Design review of the part built by this model. Coordinates are the model's own, in mm. Face numbers are marked on the shaded views. A direction names the side the tool comes from. Give positions to 0.01 mm unless a question says otherwise; leave off trailing zeros. Order: outer loops, then holes, each group sorted by start corner. A loop starts at its lowest first (then second) coordinate and runs counter-clockwise, first axis right, second up. Notation, with made-up numbers: M 78,-18.5 L 88,-18.5 A10 cw 88,-4.5 Z; hole C 23.5,-16.75 d2. An arc over 180 degrees is marked long. Answer as a JSON object with one key per item and string values.
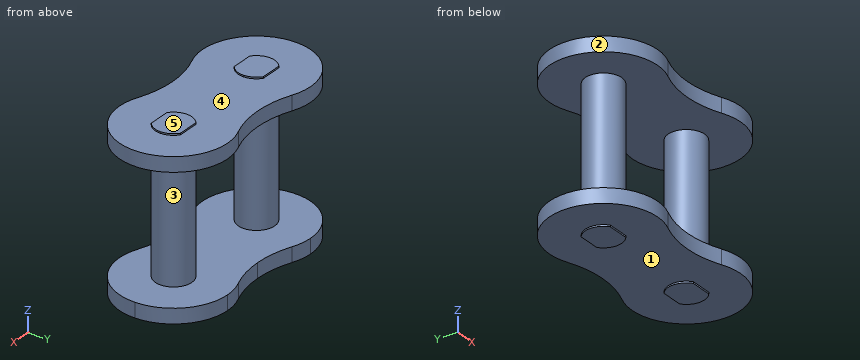
from build123d import *

# Parameters (mm, degrees)
SKETCH1_R           = 2.9718
BOSS_EXTRUDE1_DEPTH = 2.3876
SKETCH2_R           = 2.9718
BOSS_EXTRUDE2_DEPTH = 25.4
BOSS_EXTRUDE3_START = -2.3876
BOSS_EXTRUDE3_DEPTH = 2.3876
BOSS_EXTRUDE4_DEPTH = 0.254


with BuildPart() as part:
    # Sketch1 → Boss-Extrude1 (new body)
    # profile 1 of 12: a face of its own
    with BuildSketch(Plane.XY):
        with BuildLine():
            Line((-5.1181, 4.4069), (-9.525, 8.8138))
            ThreePointArc((-9.525, 8.8138), (-18.169445304, -1.71948708), (-6.152104764, -8.142889424))
            ThreePointArc((-6.152104764, -8.142889424), (-2.196593131, -4.89668492), (-0.7112, 0))
            Line((-0.7112, 0), (-5.1181, 4.4069))
        make_face()
        with Locations((-9.525, 0)):
            Circle(SKETCH1_R, mode=Mode.SUBTRACT)
    # profile 2 of 12: a face of its own
    with BuildSketch(Plane.XY):
        with BuildLine():
            ThreePointArc((-6.152104764, 8.142889424), (-7.80551292, 8.644445304), (-9.525, 8.8138))
            Line((-9.525, 8.8138), (-5.1181, 4.4069))
            Line((-5.1181, 4.4069), (-3.292702252, 6.232297748))
            ThreePointArc((-3.292702252, 6.232297748), (-4.62831508, 7.328406869), (-6.152104764, 8.142889424))
        make_face()
    # profile 3 of 12: a face of its own
    with BuildSketch(Plane.XY):
        with BuildLine():
            Line((-3.292702252, 6.232297748), (-5.1181, 4.4069))
            Line((-5.1181, 4.4069), (-0.7112, 0))
            ThreePointArc((-0.7112, 0), (-1.382110576, 3.372895236), (-3.292702252, 6.232297748))
        make_face()
    # profile 4 of 12: a face of its own
    with BuildSketch(Plane.XY):
        with BuildLine():
            ThreePointArc((-3.292702252, 6.232297748), (-1.382110576, 3.372895236), (-0.7112, 0))
            Line((-0.7112, 0), (0.7112, 0))
            ThreePointArc((0.7112, 0), (1.382110576, 3.372895236), (3.292702252, 6.232297748))
            Line((3.292702252, 6.232297748), (0, 6.232297748))
            Line((0, 6.232297748), (-3.292702252, 6.232297748))
        make_face()
    # profile 5 of 12: a face of its own
    with BuildSketch(Plane.XY):
        with BuildLine():
            ThreePointArc((-0.7112, 0), (-2.196593131, -4.89668492), (-6.152104764, -8.142889424))
            ThreePointArc((-6.152104764, -8.142889424), (0, -6.944339829), (6.152104764, -8.142889424))
            ThreePointArc((6.152104764, -8.142889424), (2.196593131, -4.89668492), (0.7112, 0))
            Line((0.7112, 0), (-0.7112, 0))
        make_face()
    # profile 6 of 12: a face of its own
    with BuildSketch(Plane.XY):
        with BuildLine():
            ThreePointArc((18.3388, 0), (15.757297748, 6.232297748), (9.525, 8.8138))
            Line((9.525, 8.8138), (5.1181, 4.4069))
            Line((5.1181, 4.4069), (0.7112, 0))
            ThreePointArc((0.7112, 0), (2.196593131, -4.89668492), (6.152104764, -8.142889424))
            ThreePointArc((6.152104764, -8.142889424), (14.42168492, -7.328406869), (18.3388, 0))
        make_face()
        with Locations((9.525, 0)):
            Circle(SKETCH1_R, mode=Mode.SUBTRACT)
    # profile 7 of 12: a face of its own
    with BuildSketch(Plane.XY):
        with BuildLine():
            Line((5.1181, 4.4069), (9.525, 8.8138))
            ThreePointArc((9.525, 8.8138), (7.80551292, 8.644445304), (6.152104764, 8.142889424))
            ThreePointArc((6.152104764, 8.142889424), (4.62831508, 7.328406869), (3.292702252, 6.232297748))
            Line((3.292702252, 6.232297748), (5.1181, 4.4069))
        make_face()
    # profile 8 of 12: a face of its own
    with BuildSketch(Plane.XY):
        with BuildLine():
            Line((0.7112, 0), (5.1181, 4.4069))
            Line((5.1181, 4.4069), (3.292702252, 6.232297748))
            ThreePointArc((3.292702252, 6.232297748), (1.382110576, 3.372895236), (0.7112, 0))
        make_face()
    # profile 9 of 12: a face of its own
    with BuildSketch(Plane.XY):
        with BuildLine():
            Line((5.1181, 4.4069), (9.525, 8.8138))
            ThreePointArc((9.525, 8.8138), (7.80551292, 8.644445304), (6.152104764, 8.142889424))
            ThreePointArc((6.152104764, 8.142889424), (4.62831508, 7.328406869), (3.292702252, 6.232297748))
            Line((3.292702252, 6.232297748), (5.1181, 4.4069))
        make_face()
    # profile 10 of 12: a face of its own
    with BuildSketch(Plane.XY):
        with BuildLine():
            ThreePointArc((6.152104764, 8.142889424), (3.133883938, 7.246767675), (0, 6.944339829))
            Line((0, 6.944339829), (0, 6.232297748))
            Line((0, 6.232297748), (3.292702252, 6.232297748))
            ThreePointArc((3.292702252, 6.232297748), (4.62831508, 7.328406869), (6.152104764, 8.142889424))
        make_face()
    # profile 11 of 12: a face of its own
    with BuildSketch(Plane.XY):
        with BuildLine():
            ThreePointArc((0, 6.944339829), (-3.133883938, 7.246767675), (-6.152104764, 8.142889424))
            ThreePointArc((-6.152104764, 8.142889424), (-4.62831508, 7.328406869), (-3.292702252, 6.232297748))
            Line((-3.292702252, 6.232297748), (0, 6.232297748))
            Line((0, 6.232297748), (0, 6.944339829))
        make_face()
    # profile 12 of 12: a face of its own
    with BuildSketch(Plane.XY):
        with BuildLine():
            ThreePointArc((-6.152104764, 8.142889424), (-7.80551292, 8.644445304), (-9.525, 8.8138))
            Line((-9.525, 8.8138), (-5.1181, 4.4069))
            Line((-5.1181, 4.4069), (-3.292702252, 6.232297748))
            ThreePointArc((-3.292702252, 6.232297748), (-4.62831508, 7.328406869), (-6.152104764, 8.142889424))
        make_face()
    extrude(amount=BOSS_EXTRUDE1_DEPTH)

    # Sketch2 → Boss-Extrude2 (add)
    with BuildSketch(Plane(origin=(0, 0, 0), x_dir=(-1, 0, 0), z_dir=(0, 0, -1))):
        with Locations((9.525, 0)):
            Circle(SKETCH2_R)
        with Locations((-9.525, 0)):
            Circle(SKETCH2_R)
    extrude(amount=-BOSS_EXTRUDE2_DEPTH)

    # Sketch3 → Boss-Extrude3 (add)
    with BuildSketch(Plane.XY.offset(25.4).offset(BOSS_EXTRUDE3_START)):
        with BuildLine():
            ThreePointArc((6.152104764, -8.142889424), (18.3388, 0), (6.152104764, 8.142889424))
            ThreePointArc((6.152104764, 8.142889424), (0, 6.944339829), (-6.152104764, 8.142889424))
            ThreePointArc((-6.152104764, 8.142889424), (-18.3388, 0), (-6.152104764, -8.142889424))
            ThreePointArc((-6.152104764, -8.142889424), (0, -6.944339829), (6.152104764, -8.142889424))
        make_face()
    extrude(amount=BOSS_EXTRUDE3_DEPTH)

    # Sketch4 → Boss-Extrude4 (add)
    with BuildSketch(Plane.XY.offset(25.4)):
        with BuildLine():
            Line((-11.302988661, -2.38125), (-7.747011339, -2.38125))
            ThreePointArc((-7.747011339, -2.38125), (-6.868364728, -1.331872467), (-6.5532, 0))
            ThreePointArc((-6.5532, 0), (-6.868364728, 1.331872467), (-7.747011339, 2.38125))
            Line((-7.747011339, 2.38125), (-11.302988661, 2.38125))
            ThreePointArc((-11.302988661, 2.38125), (-12.4968, 0), (-11.302988661, -2.38125))
        make_face()
        with BuildLine():
            ThreePointArc((7.747011339, 2.38125), (6.5532, 0), (7.747011339, -2.38125))
            Line((7.747011339, -2.38125), (11.302988661, -2.38125))
            ThreePointArc((11.302988661, -2.38125), (12.181635272, -1.331872467), (12.4968, 0))
            ThreePointArc((12.4968, 0), (12.181635272, 1.331872467), (11.302988661, 2.38125))
            Line((11.302988661, 2.38125), (7.747011339, 2.38125))
        make_face()
    boss_extrude4 = extrude(amount=BOSS_EXTRUDE4_DEPTH)

    # Mirror1: Boss-Extrude4 across plane
    add(boss_extrude4.mirror(Plane.XY.offset(12.7)))


solid = part.part
(1) Draft analysis for pull direction X (two halves, no side actions). For the marked faces 4 and 5, state which applies: +X half, -X half, draft (parallel to the pull), parting line (faces both ways), or undercut.
Checked values:
{"face 4": "undercut", "face 5": "draft"}
(2) To check wall thickness, follow L1, parallel to Z at x = -12.5, y = -4.75; L2, parallel to X at y = 2.25, z = 12; L3, parallel to X at y = 2.75, z = 1.25. State the ranges of each line that lie inside material, in increasing order. Write a range as from..to.
Checked values:
{"L1": "z = 0..2.39, 23.01..25.4", "L2": "x = -11.47..-7.58, 7.58..11.47", "L3": "x = -17.9..17.9"}
(3) We need section C-C (z = 18.5). Write out the cut boundary in (x, y) (3 decimals).
Checked values:
{"outline": "C -9.525,0 d5.944; C 9.525,0 d5.944"}
(4) We need section D-D (x = 8.5). Write out the cut boundary in (y, z).
Checked values:
{"outline": "M -8.75,0 L -2.38,0 L -2.38,-0.25 L 2.38,-0.25 L 2.38,0 L 8.75,0 L 8.75,2.39 L 2.79,2.39 L 2.79,23.01 L 8.75,23.01 L 8.75,25.4 L 2.38,25.4 L 2.38,25.65 L -2.38,25.65 L -2.38,25.4 L -8.75,25.4 L -8.75,23.01 L -2.79,23.01 L -2.79,2.39 L -8.75,2.39 Z"}
(5) We need section B-B (y = 4). Write out the cut boundary in (x, z), plus the area to 3 significant figures.
Checked values:
{"outline": "M -17.38,0 L 17.38,0 L 17.38,2.39 L -17.38,2.39 Z; M -17.38,23.01 L 17.38,23.01 L 17.38,25.4 L -17.38,25.4 Z", "area": "166 mm^2"}
(6) We need section A-A (x = -15.5). Write out the cut boundary in (y, z).
Checked values:
{"outline": "M -6.48,0 L 6.48,0 L 6.48,2.39 L -6.48,2.39 Z; M -6.48,23.01 L 6.48,23.01 L 6.48,25.4 L -6.48,25.4 Z"}
(7) Insertion check: pin 1 (8 mm diameter, centred on y = -5, z = 4.5, fed in from +X); pin 2 (6 mm diameter, centred on y = 3.5, z = 18.5, fed in from +X); pin 3 (10 mm diameter, centred on x = 4.5, z = 15, fed in from +Y). Each pin has a flat end and moves straight along its axis. Give the tip position at first contact, or say it passes through.
Checked values:
{"pin 1": "stops at x = 18.19", "pin 2": "stops at x = 12.45", "pin 3": "stops at y = 2.97"}
(8) Tool access review of the marked faces 1, 2 and 3: name each direction out of +Z, -Z, +X, -X, +Y, -Y from which nothing blocks a thin tool from reaching the whole face with its end or side.
Checked values:
{"face 1": "-Z", "face 2": "+Z, -Z", "face 3": "none"}
